from build123d import *

# Parameters (mm, degrees)
SKETCH1_W           = 100
SKETCH1_H           = 30
BOSS_EXTRUDE1_DEPTH = 3
SKETCH2_R           = 1.6
CUT_EXTRUDE1_DEPTH  = 53.28766585
SKETCH5_W           = 30
SKETCH5_H           = 30
BOSS_EXTRUDE2_DEPTH = 3
SKETCH6_R           = 1.1
CUT_EXTRUDE2_DEPTH  = 109.323589305
SKETCH7_R           = 5
CUT_EXTRUDE3_DEPTH  = 109.323589305


with BuildPart() as part:
    # Sketch1 → Boss-Extrude1 (new body)
    with BuildSketch(Plane(origin=(0, 0, 0), x_dir=(1, 0, 0), z_dir=(0, 1, 0))):
        Rectangle(SKETCH1_W, SKETCH1_H)
    extrude(amount=BOSS_EXTRUDE1_DEPTH)

    # Sketch2 → Cut-Extrude1 (cut, through all)
    with BuildSketch(Plane(origin=(0, 3, 0), x_dir=(1, 0, 0), z_dir=(0, 1, 0))):
        with Locations(Location((45, 0, 0), (0, 0, 270))):
            Circle(SKETCH2_R)
        with Locations(Location((-45, 0, 0), (0, 0, 90))):
            Circle(SKETCH2_R)
    extrude(amount=-CUT_EXTRUDE1_DEPTH, mode=Mode.SUBTRACT)

    # Sketch5 → Boss-Extrude2 (add)
    with BuildSketch(Plane(origin=(50, 0, 0), x_dir=(0, 0, -1), z_dir=(1, 0, 0))):
        with Locations((0, 15)):
            Rectangle(SKETCH5_W, SKETCH5_H)
    extrude(amount=BOSS_EXTRUDE2_DEPTH)

    # Sketch6 → Cut-Extrude2 (cut, through all)
    with BuildSketch(Plane(origin=(53, 0, 0), x_dir=(0, 0, -1), z_dir=(1, 0, 0))):
        with Locations((-6.25, 25.5)):
            Circle(SKETCH6_R)
        with Locations(Location((6.25, 25.5, 0), (0, 0, 180))):
            Circle(SKETCH6_R)
        with Locations((6.25, 4.5)):
            Circle(SKETCH6_R)
        with Locations(Location((-6.25, 4.5, 0), (0, 0, 180))):
            Circle(SKETCH6_R)
    extrude(amount=-CUT_EXTRUDE2_DEPTH, mode=Mode.SUBTRACT)

    # Sketch7 → Cut-Extrude3 (cut, through all)
    with BuildSketch(Plane(origin=(53, 0, 0), x_dir=(0, 0, -1), z_dir=(1, 0, 0))):
        with Locations((0, 15)):
            Circle(SKETCH7_R)
    extrude(amount=-CUT_EXTRUDE3_DEPTH, mode=Mode.SUBTRACT)


solid = part.part
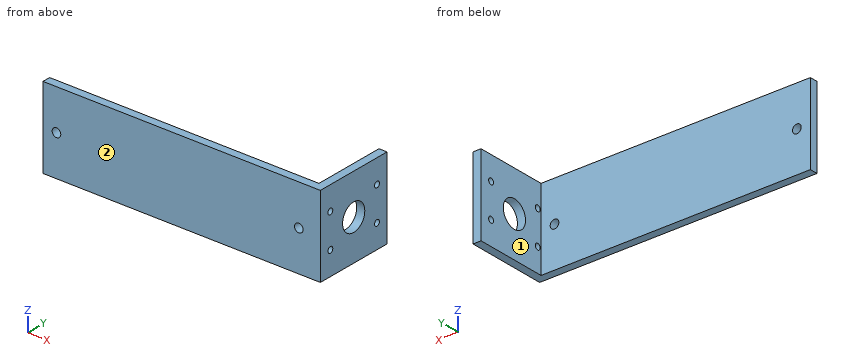
The model under review builds one solid part; all positions refer to its coordinate system, in mm. Face numbers are marked on the shaded views. A direction names the side the tool comes from. Coordinates: 2 decimals unless noted, no trailing zeros. Write each loop counter-clockwise with the first axis right and the second up, starting at its lowest first coordinate (ties: lowest second). Pieces come first, ordered by that corner, then holes. Notation, with made-up numbers: (83, 10) -> (139, 10) arc R36 ccw to (139, 49) -> close; hole circle Ø5 at (57, 61.5). An arc over 180 degrees is marked (long way). Answer in a Markdown table with one row per item.
1. We need section D-D, the plane z = 0. State the section outline as (x, y) points, and give its area (3 significant figures).
Answers below:
| item | result |
|---|---|
| outline | (-50, 0) -> (-46.6, 0) -> (-46.6, 3) -> (-50, 3) -> close; (-43.4, 0) -> (43.4, 0) -> (43.4, 3) -> (-43.4, 3) -> close; (46.6, 0) -> (53, 0) -> (53, 10) -> (50, 10) -> (50, 3) -> (46.6, 3) -> close; (50, 20) -> (53, 20) -> (53, 30) -> (50, 30) -> close |
| area | 341 mm^2 |
2. We need section A-A, the plane z = -6.25. State the section outline as (x, y) points.
Answers below:
| item | result |
|---|---|
| outline | (-50, 0) -> (53, 0) -> (53, 3.4) -> (50, 3.4) -> (50, 3) -> (-50, 3) -> close; (50, 5.6) -> (53, 5.6) -> (53, 24.4) -> (50, 24.4) -> close; (50, 26.6) -> (53, 26.6) -> (53, 30) -> (50, 30) -> close |
3. We need section B-B, the plane y = 25.5. State the section outline as (x, z) points.
Answers below:
| item | result |
|---|---|
| outline | (50, -15) -> (53, -15) -> (53, -7.35) -> (50, -7.35) -> close; (50, -5.15) -> (53, -5.15) -> (53, 5.15) -> (50, 5.15) -> close; (50, 7.35) -> (53, 7.35) -> (53, 15) -> (50, 15) -> close |
4. Clearance check with flat-ended pins moving along their axes: pin 1 Ø2 at (y, z) = (4.5, -6.25) entering from +X; pin 2 Ø1 at (y, z) = (11, -4.5) entering from -X; pin 3 Ø9 at (x, z) = (-4.5, 3.5) entering from +Y. State where each tip first meets the part, or that it passes through.
Answers below:
| item | result |
|---|---|
| pin 1 | passes through |
| pin 2 | stops at x = 50 |
| pin 3 | stops at y = 3 |
5. We need section C-C, the plane x = -45. State the section outline as (y, z) points.
Answers below:
| item | result |
|---|---|
| outline | (0, -15) -> (3, -15) -> (3, -1.6) -> (0, -1.6) -> close; (0, 1.6) -> (3, 1.6) -> (3, 15) -> (0, 15) -> close |
6. Wall thickness on probe 1 along Y at (x, z) = (51.2, -6.25); probe 2 along X at (y, z) = (9.25, -12); probe 3 along Y at (x, z) = (-30.5, -13): over which ranges is each line inside the solid? List them lowest first. Write a range as [from, to].
Answers below:
| item | result |
|---|---|
| probe 1 | y = [0, 3.4], [5.6, 24.4], [26.6, 30] |
| probe 2 | x = [50, 53] |
| probe 3 | y = [0, 3] |
7. For the marked faces 1 and 2, list the 3-axis set-ups (+Z, -Z, +X, -X, +Y, -Y) from which the entire face can be reached by the end or side of a thin tool; tool diameter is ignored.
Answers below:
| item | result |
|---|---|
| face 1 | +Z, -Z, -X, +Y |
| face 2 | +Z, -Z, +X, -X, -Y |
